from build123d import *

# Parameters (mm, degrees)
F1_DEPTH = 38.1
F2_W     = 33.8070421275
F2_H     = 20.0418584555
F3_DEPTH = 10.16
F4_R     = 5.07999
F5_R     = 1.3208962066
F5_R_2   = 1.0238880826
F6_DEPTH = 60.96


# Not quite as in the source:
# - a fillet or chamfer is up to 0.001 mm smaller than in the source, because OpenCascade refuses the exact size
# - a feature names something its author has since deleted; it is built from what else it names


with BuildPart() as f1:
    # F0 (on Front) → F1 (new body)
    with BuildSketch(Plane.XZ):
        with BuildLine():
            Line((24.7568794588, -11.2399134781), (-53.9515846949, -11.2399134781))
            Line((-53.9515846949, -11.2399134781), (-42.4472021085, -16.5292843043))
            Line((-42.4472021085, -16.5292843043), (18.5127978915, -16.5292843043))
            add(Edge.make_bspline(
                [(18.5127978915, -16.5292843043), (22.1512323361, -15.7568533336), (23.817636294, -13.7140743109), (24.7568794588, -11.2399134781)],
                knots=[0, 0, 0, 0, 7.6693401108, 7.6693401108, 7.6693401108, 7.6693401108], degree=3))
        make_face()
        with BuildLine():
            Line((-32.6618658911, 0), (-53.9515846949, -11.2399134781))
            Line((-53.9515846949, -11.2399134781), (24.7568794588, -11.2399134781))
            add(Edge.make_bspline(
                [(24.7568794588, -11.2399134781), (26.1700602844, -7.5173027852), (25.9370894642, -2.8181269591), (28.2981341089, 0)],
                knots=[7.6693401108, 7.6693401108, 7.6693401108, 7.6693401108, 19.2085929859, 19.2085929859, 19.2085929859, 19.2085929859], degree=3))
            Line((28.2981341089, 0), (-32.6618658911, 0))
        make_face()
    extrude(amount=F1_DEPTH)

    # F2 (on Top) → F3 (join)
    with BuildSketch(Plane.XY):
        with Locations((0.9121662006, -20.0837139437)):
            Rectangle(F2_W, F2_H)
    extrude(amount=F3_DEPTH)

    # F4 (radius 5.08 in the source; OpenCascade refuses exactly that, so slightly less here)
    f4_edges = [f1.edges().sort_by_distance(p)[0] for p in [
        (-15.991355, -10.062785, 5.08),
        (-15.991355, -30.104643, 5.08),
        (-15.991355, -20.083714, 0),
        (-15.991355, -20.083714, 10.16),
        (0.912166, -30.104643, 0),
        (0.912166, -10.062785, 0),
    ]]
    fillet(f4_edges, radius=F4_R)

    # F5 (on Right) → F6 (join)
    with BuildSketch(Plane.YZ):
        with Locations((-19.9000276625, 5.0683720037)):
            Circle(F5_R)
        with Locations((-19.9000276625, 5.0683720037)):
            Circle(F5_R_2, mode=Mode.SUBTRACT)
    extrude(amount=-F6_DEPTH)


solid = f1.part
Geometry: final body of the model. Coordinates: model frame, mm. A direction names the side the tool comes from. Coordinates: 2 decimals unless noted, no trailing zeros. Order: outer loops, then holes, each group sorted by start corner. A loop starts at its lowest first (then second) coordinate and runs counter-clockwise, first axis right, second up.
1) Set-up query: faces 1 (the flat face through (17.816, -20, 5)), 2 (the cylindrical face through (-38.07, -18.68, 4.56)), 3 (the flat face through (3, -10.063, 8)), 4 (the flat face through (3, -30.105, 8)). Return all of +Z, -Z, +X, -X, +Y, -Y with unobstructed straight access to the full face (end or side cutting, diameter ignored); none if empty.
Result sheet:
face 1: +Z, +X, +Y, -Y
face 2: -X
face 3: +Z, +X, -X, +Y
face 4: +Z, +X, -X, -Y
2) Draft query along Z for faces 5 (the cylindrical face through (-38.109, -20.923, 5.113)), 6 (the cylindrical face through (-17.52, -20.01, 1.45)), 7 (the cylindrical face through (3.653, -8.535, 1.449)), 8 (the flat face through (-48.28, -18.783, -13.848)). Return one class per face: released by +Z, released by -Z, zero draft, split by the parting line, or undercut.
Result sheet:
face 5: undercut
face 6: undercut
face 7: released by +Z
face 8: released by -Z
3) Section B-B (x = -44). Return loops of the section in (y, z), then the cut area to 3 significant figures.
Result sheet:
outline: (-38.1, -15.82) - (0, -15.82) - (0, -5.99) - (-38.1, -5.99) - close; circle Ø2.64 at (-19.9, 5.07); hole circle Ø2.05 at (-19.9, 5.07)
area: 377 mm2
4) First-contact query: P1, Ø8, axis at y = -13, z = -9, coming from the +X side; P2, Ø5, axis at y = -8, z = -12, coming from the +X side; P3, Ø1.8, axis at y = -19.9, z = 5.07, coming from the -X side. Flat tips, straight axial feed; report the tip coordinate or a pass-through.
Result sheet:
P1: stops at x = 26.23
P2: stops at x = 25.3
P3: stops at x = -16.07
5) Section C-C (x = -29). Return loops of the section in (y, z).
Result sheet:
outline: (-38.1, -16.53) - (0, -16.53) - (0, 0) - (-38.1, 0) - close; circle Ø2.64 at (-19.9, 5.07); hole circle Ø2.05 at (-19.9, 5.07)
6) Section A-A (x = 13). Return loops of the section in (y, z).
Result sheet:
outline: (-38.1, -16.53) - (0, -16.53) - (0, 0) - (-4.98, 0) arc R5.08 cw to (-10.06, 5.08) - (-10.06, 10.16) - (-30.1, 10.16) - (-30.1, 5.08) arc R5.08 cw to (-35.18, 0) - (-38.1, 0) - close
7) Ray query, probe 1 along Y at (x, z) = (-22.5, 5.75); probe 2 along Z at (x, y) = (-27, -23); probe 3 along Z at (x, y) = (-39.5, -5). Return the intervals inside material, ascending.
Result sheet:
probe 1: y = -21.03 to -20.66, -19.14 to -18.77
probe 2: z = -16.53 to 0
probe 3: z = -16.53 to -3.61
